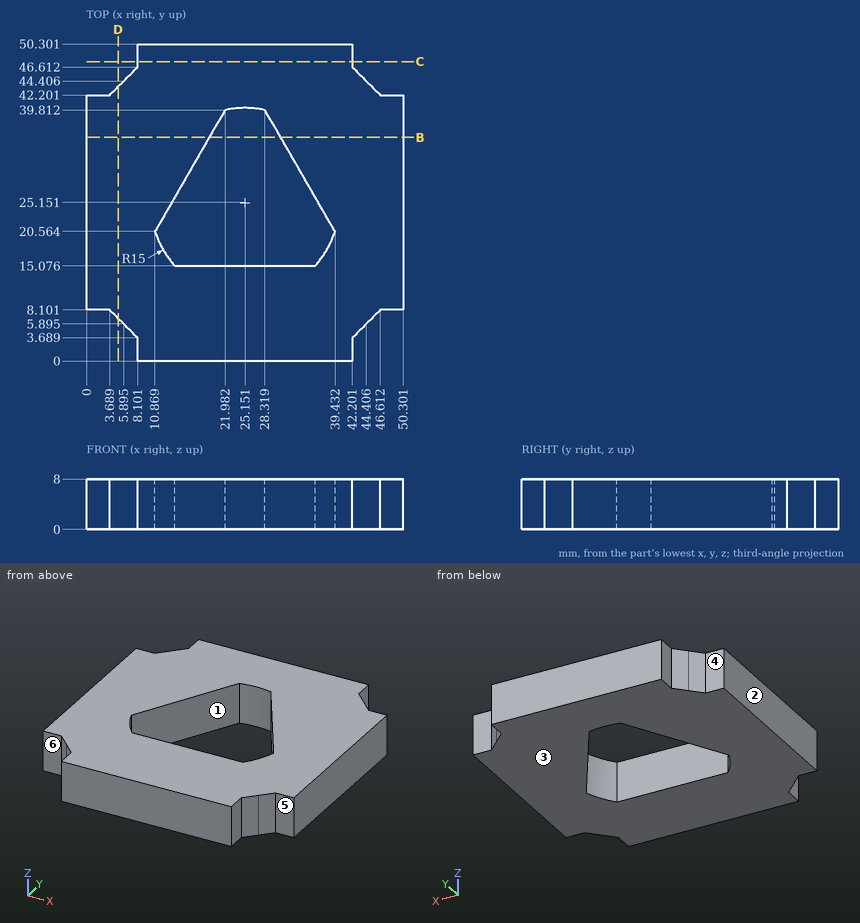
Source: three-view drawing plus pictorial views. Frame: mm from the lowest corner of the part. A direction names the side the tool comes from. Coordinates: 2 decimals unless noted, no trailing zeros. Write each loop counter-clockwise with the first axis right and the second up, starting at its lowest first coordinate (ties: lowest second). Pieces come first, ordered by that corner, then holes. Notation, with made-up numbers: (59, 85) - (87, 85) arc R36 cw to (87, 121) - close; hole circle Ø3 at (46.25, 62). An arc over 180 degrees is marked (long way). Answer as a JSON object with one key per item and string values.
Q1. Section query C-C, the plane y = 47.5. Output: boundary loops of the cut face in (x, z), plus the area to 3 significant figures.
Ans:
{"outline": "(8.1, 0) - (42.2, 0) - (42.2, 8) - (8.1, 8) - close", "area": "273 mm2"}
Q2. Draft query along X for the marked faces 1, 2 and 3. Return one class per face: released by +X, released by -X, zero draft, split by the parting line, or undercut.
Ans:
{"face 1": "undercut", "face 2": "released by -X", "face 3": "zero draft"}
Q3. Section query D-D, the plane x = 5. Output: boundary loops of the cut face in (y, z), plus the area to 3 significant figures.
Ans:
{"outline": "(6.79, 0) - (43.51, 0) - (43.51, 8) - (6.79, 8) - close", "area": "294 mm2"}
Q4. Material intervals for line 1 (Y direction, x = 25.5, z = 4.25) (1 decimal); line 2 (Y direction, x = 27, z = 3.25) (1 decimal); line 3 (X direction, y = 21.5, z = 7.25), sorted ascending. Write a range as [from, to].
Ans:
{"line 1": "y = [0, 15.1], [40.1, 50.3]", "line 2": "y = [0, 15.1], [40, 50.3]", "line 3": "x = [0, 11.41], [38.89, 50.3]"}
Q5. Set-up query: the marked faces 4, 5 and 6. Return all of +Z, -Z, +X, -X, +Y, -Y with unobstructed straight access to the full face (end or side cutting, diameter ignored); none if empty.
Ans:
{"face 4": "+Z, -Z, -X, +Y", "face 5": "+Z, -Z, +X, -Y", "face 6": "+Z, -Z, -X, -Y"}
Q6. First-contact query: pin 1 Ø3 at (x, z) = (1.5, 3) entering from +Y; pin 2 Ø1.1 at (x, z) = (1, 4.5) entering from -Y; pin 3 Ø4 at (y, z) = (48, 4.5) entering from -X. Flat tips, straight axial feed; report the tip coordinate or a pass-through.
Ans:
{"pin 1": "stops at y = 42.2", "pin 2": "stops at y = 8.1", "pin 3": "stops at x = 7.49"}
Q7. Section query B-B, the plane y = 35.5. Output: boundary loops of the cut face in (x, z).
Ans:
{"outline": "(0, 0) - (19.49, 0) - (19.49, 8) - (0, 8) - close; (30.81, 0) - (50.3, 0) - (50.3, 8) - (30.81, 8) - close"}
